Here's how the part is built. I have some questions about the finished solid (model axes, mm). A direction names the side the tool comes from. Round coordinates to 2 decimals unless told otherwise and drop trailing zeros. Order: outer loops, then holes, each group sorted by start corner. A loop starts at its lowest first (then second) coordinate and runs counter-clockwise, first axis right, second up. Notation, with made-up numbers: (48, 6) -> (72, 6) arc R27 cw to (72, 25) -> close; hole circle Ø2 at (23, 28.5). An arc over 180 degrees is marked (long way). One line per item, written item: value.
```python
from build123d import *

# Parameters (mm, degrees)
SKETCH1_W           = 90
SKETCH1_H           = 90
SKETCH1_R           = 2.2
SKETCH1_R_2         = 13
BOSS_EXTRUDE1_DEPTH = 5
SKETCH1_3_R         = 13
SKETCH1_3_R_2       = 9.6
SKETCH1_3_R_3       = 8.6
SKETCH1_3_R_4       = 6
BOSS_EXTRUDE2_DEPTH = 3
SKETCH1_4_R         = 13
SKETCH1_4_R_2       = 9.6
SKETCH1_4_R_3       = 8.6
BOSS_EXTRUDE3_DEPTH = 8
SKETCH1_5_R         = 13
SKETCH1_5_R_2       = 9.6
BOSS_EXTRUDE4_DEPTH = 10
CHAMFER1_SIZE       = 4


with BuildPart() as part:
    # Sketch1 → Boss-Extrude1 (new body)
    with BuildSketch(Plane(origin=(0, 0, 0), x_dir=(1, 0, 0), z_dir=(0, 1, 0))):
        Rectangle(SKETCH1_W, SKETCH1_H)
        with Locations(Location((-35, -35, 0), (0, 0, 270))):
            Circle(SKETCH1_R, mode=Mode.SUBTRACT)
        with Locations(Location((35, -35, 0), (0, 0, 270))):
            Circle(SKETCH1_R, mode=Mode.SUBTRACT)
        with Locations(Location((35, 35, 0), (0, 0, 270))):
            Circle(SKETCH1_R, mode=Mode.SUBTRACT)
        with Locations(Location((-35, 35, 0), (0, 0, 270))):
            Circle(SKETCH1_R, mode=Mode.SUBTRACT)
        with Locations(Location((0, 0, 0), (0, 0, 270))):
            Circle(SKETCH1_R_2, mode=Mode.SUBTRACT)
    extrude(amount=BOSS_EXTRUDE1_DEPTH)

    # Sketch1_3 → Boss-Extrude2 (add)
    # profile 1 of 3: a face of its own
    with BuildSketch(Plane(origin=(0, 0, 0), x_dir=(1, 0, 0), z_dir=(0, 1, 0))):
        with Locations(Location((0, 0, 0), (0, 0, 270))):
            Circle(SKETCH1_3_R)
        Circle(SKETCH1_3_R_2, mode=Mode.SUBTRACT)
    # profile 2 of 3: a face of its own
    with BuildSketch(Plane(origin=(0, 0, 0), x_dir=(1, 0, 0), z_dir=(0, 1, 0))):
        Circle(SKETCH1_3_R_2)
        Circle(SKETCH1_3_R_3, mode=Mode.SUBTRACT)
    # profile 3 of 3: a face of its own
    with BuildSketch(Plane(origin=(0, 0, 0), x_dir=(1, 0, 0), z_dir=(0, 1, 0))):
        Circle(SKETCH1_3_R_3)
        with Locations(Location((0, 0, 0), (0, 0, 270))):
            Circle(SKETCH1_3_R_4, mode=Mode.SUBTRACT)
    extrude(amount=BOSS_EXTRUDE2_DEPTH)

    # Sketch1_4 → Boss-Extrude3 (add)
    # profile 1 of 2: a face of its own
    with BuildSketch(Plane(origin=(0, 0, 0), x_dir=(1, 0, 0), z_dir=(0, 1, 0))):
        with Locations(Location((0, 0, 0), (0, 0, 270))):
            Circle(SKETCH1_4_R)
        Circle(SKETCH1_4_R_2, mode=Mode.SUBTRACT)
    # profile 2 of 2: a face of its own
    with BuildSketch(Plane(origin=(0, 0, 0), x_dir=(1, 0, 0), z_dir=(0, 1, 0))):
        Circle(SKETCH1_4_R_2)
        with Locations(Location((0, 0, 0), (0, 0, 270))):
            Circle(SKETCH1_4_R_3, mode=Mode.SUBTRACT)
    extrude(amount=BOSS_EXTRUDE3_DEPTH)

    # Sketch1_5 → Boss-Extrude4 (add)
    with BuildSketch(Plane(origin=(0, 0, 0), x_dir=(1, 0, 0), z_dir=(0, 1, 0))):
        with Locations(Location((0, 0, 0), (0, 0, 270))):
            Circle(SKETCH1_5_R)
        with Locations(Location((0, 0, 0), (0, 0, 270))):
            Circle(SKETCH1_5_R_2, mode=Mode.SUBTRACT)
    extrude(amount=BOSS_EXTRUDE4_DEPTH)

    # Chamfer1
    chamfer1_edges = [part.edges().sort_by_distance(p)[0] for p in [
        (-45, 2.5, 45),
        (-45, 2.5, -45),
        (45, 2.5, -45),
        (45, 2.5, 45),
    ]]
    chamfer(chamfer1_edges, length=CHAMFER1_SIZE)


solid = part.part
```
Q1. If we mould it in two halves opening along X, with no side actions, what happens to faces 3 (the face through (32.852, 2.465, -35.477)), 4 (the face through (11, 0, -1)), 5 (the face through (45, 2, 1))? For each: pulls with the +X half, pulls with the -X half, needs draft (parallel to the pull), parting line crosses it, or undercut.
Answers:
face 3: undercut
face 4: needs draft
face 5: pulls with the +X half
Q2. I want a section at D-D on x = 4.5. Write out the boundary of the cut face in (y, z).
Answers:
outline: (0, -45) -> (5, -45) -> (5, -12.2) -> (10, -12.2) -> (10, -8.48) -> (8, -8.48) -> (8, -7.33) -> (3, -7.33) -> (3, -3.97) -> (0, -3.97) -> close; (0, 3.97) -> (3, 3.97) -> (3, 7.33) -> (8, 7.33) -> (8, 8.48) -> (10, 8.48) -> (10, 12.2) -> (5, 12.2) -> (5, 45) -> (0, 45) -> close
Q3. I want a section at C-C on z = -35. Write out the boundary of the cut face in (x, y).
Answers:
outline: (-45, 0) -> (-37.2, 0) -> (-37.2, 5) -> (-45, 5) -> close; (-32.8, 0) -> (32.8, 0) -> (32.8, 5) -> (-32.8, 5) -> close; (37.2, 0) -> (45, 0) -> (45, 5) -> (37.2, 5) -> close
Q4. Which directions (+Z, -Z, +X, -X, +Y, -Y) give clear straight access to the entire face, cutting with the end or side of a thin tool? Please do faces 1 (the face through (-5.233, 5.465, -6.825)), 2 (the face through (-1, 2, 45)).
Answers:
face 1: +Y
face 2: +Z, +X, -X, +Y, -Y
Q5. For P1, Ø5, axis at x = 0.5, z = -4, coming from the +Y side; P2, Ø4, axis at x = 24, z = 29, coming from the +Y side; P3, Ø3.5, axis at x = -35, z = 35, coming from the +Y side; P4, Ø6, axis at x = -0.5, z = -6, coming from the +Y side, each with a flat end and sliding along its axis, tell me the tip position at first contact or that it passes through.
Answers:
P1: y = 3
P2: y = 5
P3: through
P4: y = 8
Q6. I want a section at B-B on x = -35. Write out the boundary of the cut face in (y, z).
Answers:
outline: (0, -45) -> (5, -45) -> (5, -37.2) -> (0, -37.2) -> close; (0, -32.8) -> (5, -32.8) -> (5, 32.8) -> (0, 32.8) -> close; (0, 37.2) -> (5, 37.2) -> (5, 45) -> (0, 45) -> close
Q7. I want a section at A-A on z = 0. Write out the boundary of the cut face in (x, y), then the cut area to 3 significant figures.
Answers:
outline: (-45, 0) -> (-6, 0) -> (-6, 3) -> (-8.6, 3) -> (-8.6, 8) -> (-9.6, 8) -> (-9.6, 10) -> (-13, 10) -> (-13, 5) -> (-45, 5) -> close; (6, 0) -> (45, 0) -> (45, 5) -> (13, 5) -> (13, 10) -> (9.6, 10) -> (9.6, 8) -> (8.6, 8) -> (8.6, 3) -> (6, 3) -> close
area: 420 mm2
Q8. I need wall thicknesses on line 1 along X through (y, z) = (1, 35); line 2 along X through (y, z) = (9.4, 0); line 3 along Y through (x, z) = (27.5, -5.5). Which ranges of each line are inside material? Lowest first, please.
Answers:
line 1: -45 to -37.2, -32.8 to 32.8, 37.2 to 45
line 2: -13 to -9.6, 9.6 to 13
line 3: 0 to 5
